Autodesk Inventor part; units mm, degrees
ref_plane "XZ Plane" through (0, 0, 0) normal (0, 1, 0) x (-1, 0, 0)
sketch "Sketch1" plane through (0, 0, 0) normal (0, 0, 1) x (1, 0, 0)
  line L0 (-2.05, 2.05) -> (2.05, 2.05)
  line L1 (2.05, 2.05) -> (2.05, -2.05)
  line L2 (2.05, -2.05) -> (-2.05, -2.05)
  line L3 (-2.05, -2.05) -> (-2.05, 2.05)
  line L4 (0, 2.05) -> (0, -2.05) construction
  line L5 (0, 7.5) -> (-15.55, 7.5)
  line L6 (-15.55, 7.5) -> (-15.55, 6)
  line L7 (-15.55, 6) -> (-3.55, 6)
  line L8 (-3.55, 6) -> (-3.55, -6)
  line L9 (-3.55, -6) -> (-15.55, -6)
  line L10 (-15.55, -6) -> (-15.55, -7.5)
  line L11 (-15.55, -7.5) -> (-0.55, -7.5)
  line L12 (-2.05, 0) -> (2.05, 0) construction
  line L13 (0, 7.5) -> (15.55, 7.5)
  line L14 (15.55, 7.5) -> (15.55, 6)
  line L15 (15.55, 6) -> (3.55, 6)
  line L16 (3.55, 6) -> (3.55, -6)
  line L17 (3.55, -6) -> (15.55, -6)
  line L18 (15.55, -6) -> (15.55, -7.5)
  line L19 (15.55, -7.5) -> (-0.55, -7.5)
  line L20 (-2.05, 2.05) -> (2.05, -2.05) construction
  line L21 (2.05, 2.05) -> (-2.05, -2.05) construction
  line L22 (0, 7.5) -> (0, 2.05) construction
  point P0 (0, 0)
  point P1 (0, 0)
  point P2 (0, 0)
  dimension "d3" = 4.1
  dimension "d4" = 4.1
  dimension "d5" = 12
  dimension "d6" = 1.5
  dimension "d7" = 1.5
  dimension "d8" = 5.45
  dimension "d9" = 5.45
  dimension "d10" = 1.5
  dimension "d11" = 12
  dimension "d37" = 15
extrude "Extrusion1" add sketch "Sketch1" along normal blind 10
sketch "Sketch5" plane through (0, 0, 10) normal (0, 0, 1) x (1, 0, 0)
  line L0 (6, 19.5) -> (7.5, 19.5)
  line L1 (7.5, 19.5) -> (7.5, 7.5)
  line L2 (7.5, 7.5) -> (6, 7.5)
  line L3 (6, 7.5) -> (6, 19.5)
  line L4 (15.55, 7.5) -> (-15.55, 7.5)
  line L5 (3.55, -6) -> (3.55, 6)
  line L6 (0, 0) -> (0, 23.4065) construction
  dimension "d41" = 1.5
  dimension "d42" = 12
  dimension "d47" = 6
extrude "Extrusion5" add sketch "Sketch5" against normal up to surface (10 mm away)
mirror "Mirror1" about plane through (0, 0, 0) normal (1, 0, 0) of "Extrusion5"
fillet "Fillet1" radius 3 2 edges at (-7.5, 7.5, 5) (7.5, 7.5, 5)
fillet "Fillet2" radius 0.5 6 edges at (-3.55, 6, 5) (-3.55, -6, 5) (3.55, -6, 5) (3.55, 6, 5) (-6, 7.5, 5) (6, 7.5, 5)
fillet "Fillet3" radius 2 12 edges at (-6.75, 19.5, 10) (-15.55, 6.75, 10) (-6.75, 19.5, 0) (6.75, 19.5, 0) (6.75, 19.5, 10) (15.55, 6.75, 10) (15.55, 6.75, 0) (15.55, -6.75, 0) (15.55, -6.75, 10) (-15.55, -6.75, 10) (-15.55, -6.75, 0) (-15.55, 6.75, 0)
sketch "Sketch7" plane through (0, 0, 0) normal (0, 0, -1) x (-1, 0, 0)
  line L0 (-2.05, 5.05) -> (2.05, 5.05)
  line L1 (2.05, 5.05) -> (2.05, 3.55)
  line L2 (2.05, 3.55) -> (-2.05, 3.55)
  line L3 (-2.05, 3.55) -> (-2.05, 5.05)
  line L4 (-2.05, -3.55) -> (2.05, -3.55)
  line L5 (2.05, -3.55) -> (2.05, -5.05)
  line L6 (2.05, -5.05) -> (-2.05, -5.05)
  line L7 (-2.05, -5.05) -> (-2.05, -3.55)
  line L8 (2.05, 2.05) -> (-2.05, 2.05)
  line L9 (-2.05, -2.05) -> (2.05, -2.05)
  line L10 (2.05, -2.05) -> (2.05, 2.05)
  line L11 (-2.05, 2.05) -> (-2.05, -2.05)
  point P0 (0, 0)
  dimension "d55" = 1.5
  dimension "d56" = 1.5
  dimension "d57" = 1.5
  dimension "d58" = 1.5
extrude "Extrusion7" cut sketch "Sketch7" against normal blind 10 contours L0 L1 L2 L3 | L4 L5 L6 L7
equation "\"d7\" = d6"
equation "\"d8\" = d9"
properties part number "fuselage_tail_interface_airfoiled" material "ABS Plastic"
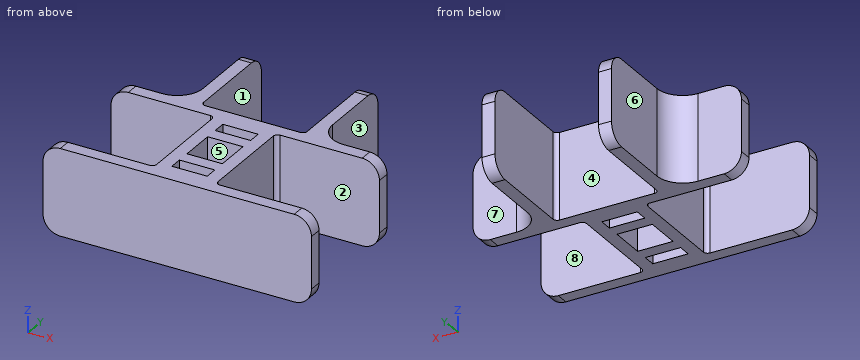
Geometry: final body of the model. Coordinates: model frame, mm. Face numbers are marked on the shaded views. A direction names the side the tool comes from. Give positions to 0.01 mm unless a question says otherwise; leave off trailing zeros. Write each loop counter-clockwise with the first axis right and the second up, starting at its lowest first coordinate (ties: lowest second). Pieces come first, ordered by that corner, then holes. Notation, with made-up numbers: (-19, 67.25) -> (16, 67.25) arc R30 cw to (16, 91.25) -> close; hole circle Ø1 at (41, 35). An arc over 180 degrees is marked (long way). Answer in a Markdown table with one row per item.
(1) Set-up query: the marked faces 4, 5, 6, 7 and 8. Return all of +Z, -Z, +X, -X, +Y, -Y with unobstructed straight access to the full face (end or side cutting, diameter ignored); none if empty.
Answers below:
| item | result |
|---|---|
| face 4 | +Z, -Z, +Y |
| face 5 | +Z, -Z |
| face 6 | +Z, -Z, -X, +Y |
| face 7 | +Z, -Z, +X, +Y |
| face 8 | +Z, -Z, +X |
(2) Section query B-B on y = 1. Return loops of the section in (x, z), then the cut area to 3 significant figures.
Answers below:
| item | result |
|---|---|
| outline | (-3.55, 0) -> (-2.05, 0) -> (-2.05, 10) -> (-3.55, 10) -> close; (2.05, 0) -> (3.55, 0) -> (3.55, 10) -> (2.05, 10) -> close |
| area | 30.0 mm^2 |
(3) Draft query along X for the marked faces 1, 2 and 3. Return one class per face: +X half, -X half, draft (parallel to the pull), parting line (faces both ways), or undercut.
Answers below:
| item | result |
|---|---|
| face 1 | undercut |
| face 2 | draft |
| face 3 | +X half |
(4) Pin query (flat end, axial travel): pin 1 (3 mm diameter, centred on y = 11, z = 4, fed in from +X); pin 2 (1.5 mm diameter, centred on x = 12, z = 2.5, fed in from +Y); pin 3 (0.8 mm diameter, centred on y = -4, z = 4.5, fed in from -X). Return the tip coordinate at first contact, or that it passes through.
Answers below:
| item | result |
|---|---|
| pin 1 | x = 7.67 |
| pin 2 | y = 7.5 |
| pin 3 | x = -3.55 |
(5) Ray query, line 1 along Y through (x, z) = (12.5, 3.75); line 2 along Y through (x, z) = (-1.5, 8.5). Return the intervals inside material, ascending. Write a range as [from, to].
Answers below:
| item | result |
|---|---|
| line 1 | [-7.5, -6], [6, 7.5] |
| line 2 | [-7.5, -5.05], [-3.55, -2.05], [2.05, 3.55], [5.05, 7.5] |
(6) Section query C-C on z = 5. State how many separate pieces and enclosed holes the cut face has, then the cut area to 3 significant figures.
Answers below:
| item | result |
|---|---|
| separate pieces | 1 |
| enclosed holes | 3 |
| area | 190 mm^2 |
(7) Section query A-A on x = 11. Return loops of the section in (y, z).
Answers below:
| item | result |
|---|---|
| outline | (-7.5, 0) -> (-6, 0) -> (-6, 10) -> (-7.5, 10) -> close; (6, 0) -> (7.5, 0) -> (7.5, 10) -> (6, 10) -> close |
